from build123d import *

# Parameters (mm, degrees)
SALIENTE_EXTRUIR1_DEPTH = 6.35
CROQUIS2_W              = 152.4
CROQUIS2_H              = 6.35
CORTAR_EXTRUIR1_DEPTH   = 6.35
CROQUIS3_R              = 6.35
CORTAR_EXTRUIR2_DEPTH   = 6.35
CROQUIS4_R              = 6.35
CORTAR_EXTRUIR3_DEPTH   = 6.35
REDONDEO1_R             = 25.4
CROQUIS5_W              = 3.81
CROQUIS5_H              = 196.85
CORTAR_EXTRUIR4_DEPTH   = 6.35


with BuildPart() as part:
    # Croquis1 → Saliente-Extruir1 (new body)
    with BuildSketch(Plane.XY):
        with BuildLine():
            Line((6.35, 165.1), (311.15, 165.1))
            Line((311.15, 165.1), (311.15, -165.1))
            Line((311.15, -165.1), (-311.15, -165.1))
            Line((-311.15, -165.1), (-311.15, 165.1))
            ThreePointArc((-311.15, 165.1), (-152.4, 230.856403027), (6.35, 165.1))
        make_face()
    extrude(amount=SALIENTE_EXTRUIR1_DEPTH)

    # Croquis2 → Cortar-Extruir1 (cut)
    with BuildSketch(Plane.XY.offset(6.35)):
        with Locations((152.4, 60.325)):
            Rectangle(CROQUIS2_W, CROQUIS2_H)
    extrude(amount=-CORTAR_EXTRUIR1_DEPTH, mode=Mode.SUBTRACT)

    # Croquis3 → Cortar-Extruir2 (cut)
    with BuildSketch(Plane.XY.offset(6.35)):
        with Locations((-152.4, 133.35)):
            Circle(CROQUIS3_R)
        with Locations((-215.9, 133.35)):
            Circle(CROQUIS3_R)
        with Locations((-88.9, 133.35)):
            Circle(CROQUIS3_R)
    extrude(amount=-CORTAR_EXTRUIR2_DEPTH, mode=Mode.SUBTRACT)

    # Croquis4 → Cortar-Extruir3 (cut)
    with BuildSketch(Plane.XY.offset(6.35)):
        with Locations((-273.05, 165.1)):
            Circle(CROQUIS4_R)
        with Locations((-31.75, 165.1)):
            Circle(CROQUIS4_R)
    extrude(amount=-CORTAR_EXTRUIR3_DEPTH, mode=Mode.SUBTRACT)

    # Redondeo1
    redondeo1_edges = [part.edges().sort_by_distance(p)[0] for p in [
        (311.15, 165.1, 3.175),
    ]]
    fillet(redondeo1_edges, radius=REDONDEO1_R)

    # Croquis5 → Cortar-Extruir4 (cut)
    with BuildSketch(Plane.XY.offset(6.35)):
        with Locations((-306.705, -60.325)):
            Rectangle(CROQUIS5_W, CROQUIS5_H)
        with Locations((306.705, -60.325)):
            Rectangle(CROQUIS5_W, CROQUIS5_H)
    extrude(amount=-CORTAR_EXTRUIR4_DEPTH, mode=Mode.SUBTRACT)


solid = part.part
Design review of the part built by this model. Coordinates are the model's own, in mm. Round coordinates to 2 decimals unless told otherwise and drop trailing zeros. Loops run counter-clockwise (first coordinate to the right, second up) from the corner with the lowest first, then second, coordinate; pieces in that order, holes last. Notation, with made-up numbers: (38.5, 6) - (44.5, 6) arc R20 ccw to (44.5, 18) - close; hole circle Ø3 at (-4, -13.5). An arc over 180 degrees is marked (long way). One line per question, with ' | ' between items.
1. We need section D-D, the plane x = -273.05. State the section outline as (y, z) points, and give its area (3 significant figures).
Results are:
outline: (-165.1, 0) - (158.75, 0) - (158.75, 6.35) - (-165.1, 6.35) - close; (171.45, 0) - (195.68, 0) - (195.68, 6.35) - (171.45, 6.35) - close | area: 2,210 mm²
2. Clearance check with flat-ended pins moving along their axes: P1, Ø2, axis at x = 90, z = 5, coming from the +Y side; P2, Ø2, axis at x = -194.5, z = 4.5, coming from the +Y side; P3, Ø10, axis at x = -152.4, y = 133.35, coming from the -Z side; P4, Ø2, axis at y = 150.5, z = 5.5, coming from the +X side. State where each tip first meets the part, or that it passes through.
Results are:
P1: stops at y = 165.1 | P2: stops at y = 227.06 | P3: passes through | P4: stops at x = 309.18
3. We need section A-A, the plane x = -152.4. State the section outline as (y, z) points.
Results are:
outline: (-165.1, 0) - (127, 0) - (127, 6.35) - (-165.1, 6.35) - close; (139.7, 0) - (230.86, 0) - (230.86, 6.35) - (139.7, 6.35) - close
4. We need section B-B, the plane z = 4.75. State how many separate pieces and enclosed holes the cut face has, and give its area (3 significant figures).
Results are:
separate pieces: 1 | enclosed holes: 8 | area: 217,000 mm²
5. For L1, parallel to X at y = -82.5, z = 6; L2, parallel to Y at x = 50, z = 3.25; L3, parallel to Y at x = -215.9, z = 3, list the stretches that pass through material, from the lowest coordinate up. Write a range as [from, to].
Results are:
L1: x = [-311.15, -308.61], [-304.8, 304.8], [308.61, 311.15] | L2: y = [-165.1, 165.1] | L3: y = [-165.1, 127], [139.7, 221.69]
6. Draft analysis for pull direction X (two halves, no side actions). For faces 1 (the face through (-154.869, 230.843, 3.131)), 2 (the face through (-33.13, 158.9, 3.22)), 3 (the face through (-146.534, 130.918, 3.219)), 4 (the face through (303.51, 157.86, 3.22)), state which applies: released by +X, released by -X, zero draft, split by the parting line, or undercut.
Results are:
face 1: split by the parting line | face 2: undercut | face 3: undercut | face 4: released by +X
7. We need section C-C, the plane y = 133.35. State the section outline as (x, z) points.
Results are:
outline: (-311.15, 0) - (-222.25, 0) - (-222.25, 6.35) - (-311.15, 6.35) - close; (-209.55, 0) - (-158.75, 0) - (-158.75, 6.35) - (-209.55, 6.35) - close; (-146.05, 0) - (-95.25, 0) - (-95.25, 6.35) - (-146.05, 6.35) - close; (-82.55, 0) - (311.15, 0) - (311.15, 6.35) - (-82.55, 6.35) - close
